from build123d import *

# Parameters (mm, degrees)
F0_R            = 16
F1_DEPTH        = 7.9
F2_R            = 8.11
F3_DEPTH        = 3.8
F4_R            = 6
F5_DEPTH        = 7.901
F6_R            = 1.55
F7_DEPTH        = 7.901
F7_COPIES_COUNT = 6
F8_R            = 8
F8_R_2          = 6
F9_DEPTH        = 2
F10_SIZE2       = 2.10999
F10_SIZE        = 2.10999


# Not quite as in the source:
# - a fillet or chamfer is up to 0.001 mm smaller than in the source, because OpenCascade refuses the exact size
# - a pattern or mirror of a feature is missing from the dataset's text; its kind, count and spacing are read off the source's solid


with BuildPart() as f1:
    # F0 (on Right) → F1 (new body)
    with BuildSketch(Plane.YZ):
        Circle(F0_R)
    extrude(amount=F1_DEPTH)

    # F2 (on face) → F3 (cut)
    with BuildSketch(Plane(origin=(0, 0, 0), x_dir=(0, -1, 0), z_dir=(-1, 0, 0))):
        Circle(F2_R)
    extrude(amount=-F3_DEPTH, mode=Mode.SUBTRACT)

    # F4 (on face) → F5 (cut, through all)
    with BuildSketch(Plane.YZ.offset(7.9)):
        Circle(F4_R)
    extrude(amount=-F5_DEPTH, mode=Mode.SUBTRACT)

    # F6 (on face) → F7 (cut, through all)
    with BuildSketch(Plane(origin=(0, 0, 0), x_dir=(0, -1, 0), z_dir=(-1, 0, 0))):
        with Locations((-3.4491492906, 12.0147146937)):
            Circle(F6_R)
    f7 = extrude(amount=-F7_DEPTH, mode=Mode.SUBTRACT)

    # F7_copies: F7 ×6 about axis
    f7_copies_axis = Axis((0, 0, 0), (1, 0, 0))
    for i in range(1, F7_COPIES_COUNT):
        add(f7.rotate(f7_copies_axis, i * 360 / F7_COPIES_COUNT), mode=Mode.SUBTRACT)

    # F8 (on face) → F9 (join)
    with BuildSketch(Plane.YZ.offset(7.9)):
        Circle(F8_R)
        Circle(F8_R_2, mode=Mode.SUBTRACT)
    extrude(amount=F9_DEPTH)

    # F10 (size 2.11 and 2.11 in the source; OpenCascade refuses exactly that, so slightly less here)
    f10_edges = [f1.edges().sort_by_distance(p)[0] for p in [
        (3.8, -6, 0),
    ]]
    chamfer(f10_edges, length=F10_SIZE, length2=F10_SIZE2)


solid = f1.part
CAD build for the part. Positions are in the model's coordinates, mm. A direction names the side the tool comes from. Round coordinates to 2 decimals unless told otherwise and drop trailing zeros. Write each loop counter-clockwise with the first axis right and the second up, starting at its lowest first coordinate (ties: lowest second). Pieces come first, ordered by that corner, then holes. Notation, with made-up numbers: M 58,29.25 L 91,29.25 A22 cw 91,65.25 Z; hole C -27.5,-37 d3. An arc over 180 degrees is marked long. Use a Markdown table: item, result. Add a question column.
1. Slice it at C-C on x = 2.5. Give the cut face in (y, z), then the cut area to 3 significant figures.
2. Slice it at D-D on x = 9. Give the cut face in (y, z), then the cut area to 3 significant figures.
3. 3-axis set-ups, long thin cutter, end or side, ignore diameter. For faces 1 (the face through (1.87, -7.49, -3.11)), 2 (the face through (0, 7, -7)): which of +Z, -Z, +X, -X, +Y, -Y reach the whole face in a straight line?
4. Flat gauge pins, fed straight in: P1, Ø9.5, axis at y = 0, z = 0, coming from the -X side; P2, Ø1, axis at x = 5.5, z = -2.5, coming from the -Y side. Where does each tip first touch, or does it go through?
5. Pull direction Z, two halves, no side cores. Call faces 3 (the face through (7.9, -3.8, 7.3)), 4 (the face through (8.89, -1.73, -7.81)), 5 (the face through (3.895, 2.616, 13.322)): released by +Z, released by -Z, zero draft, split by the parting line, or undercut.
6. Drill centre lines: probe 1 along Y at (x, z) = (3.5, 2.5); probe 2 along Y at (x, z) = (1.25, -4); probe 3 along Y at (x, z) = (7.75, 12). Where is each one in solid material? Low to high.
Reply:
| question | item | result |
|---|---|---|
| 1 | outline | C 0,0 d32; hole C -12.13,-3.02 d3.1; hole C -8.68,8.99 d3.1; hole C 0,0 d16.22; hole C -3.45,-12.01 d3.1; hole C 3.45,12.01 d3.1; hole C 8.68,-8.99 d3.1; hole C 12.13,3.02 d3.1 |
| 1 | area | 552 mm^2 |
| 2 | outline | C 0,0 d16; hole C 0,0 d12 |
| 2 | area | 88.0 mm^2 |
| 3 | face 1 | -X |
| 3 | face 2 | +Z, -Z, -X, +Y, -Y |
| 4 | P1 | passes through |
| 4 | P2 | stops at y = -15.87 |
| 5 | face 3 | zero draft |
| 5 | face 4 | split by the parting line |
| 5 | face 5 | undercut |
| 6 | probe 1 | y = -15.8 to -7.72, 7.72 to 10.67, 13.59 to 15.8 |
| 6 | probe 2 | y = -15.49 to -13.33, -10.93 to -7.05, 7.05 to 15.49 |
| 6 | probe 3 | y = -10.58 to 1.9, 5 to 10.58 |
